Check sheet for the drawn part. Datum: minimum x, y, z corner. Units: mm. Give positions to 0.01 mm unless a question says otherwise; leave off trailing zeros. Write each loop counter-clockwise with the first axis right and the second up, starting at its lowest first coordinate (ties: lowest second). Pieces come first, ordered by that corner, then holes.
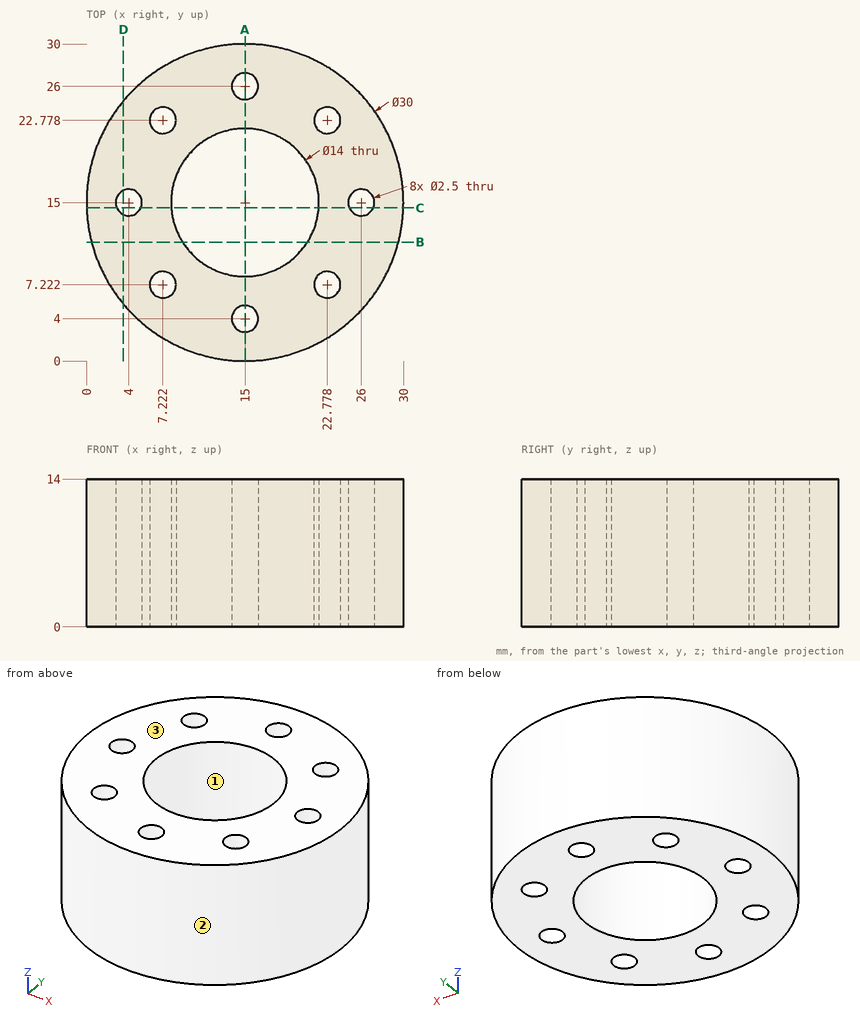
1) Sectioned sample at D-D on x = 3.5. Record the boundary of the cut face in (y, z).
2) Sectioned sample at C-C on y = 14.5. Record the boundary of the cut face in (x, z).
3) Sectioned sample at A-A on x = 15. Record the boundary of the cut face in (y, z), then the cut area to 3 significant figures.
4) Gauge pin test, flat ends, axial feed: pin 1 (2 mm diameter, centred on x = 4, y = 15, fed in from -Z); pin 2 (3 mm diameter, centred on y = 9.5, z = 9, fed in from -X); pin 3 (6 mm diameter, centred on y = 5, z = 1.5, fed in from +X); pin 4 (8 mm diameter, centred on y = 27, z = 11, fed in from -X). Record the tip position at first contact, or that the pin passes through.
5) Sectioned sample at B-B on y = 11.25. Record the boundary of the cut face in (x, z), then the cut area to 3 significant figures.
6) Scan lines: L1, parallel to Y at x = 15, z = 5; L2, parallel to Y at x = 7.5, z = 5.5; L3, parallel to X at y = 23, z = 9.75. Record each from-to range of solid material in increasing order.
7) Draft check along X on the marked faces 1, 2 and 3. Enter one of: +X half, -X half, draft (parallel to the pull), parting line (faces both ways), or undercut.
Answers below:
1. outline: (5.37, 0) - (13.85, 0) - (13.85, 14) - (5.37, 14) - close; (16.15, 0) - (24.63, 0) - (24.63, 14) - (16.15, 14) - close
2. outline: (0.01, 0) - (2.85, 0) - (2.85, 14) - (0.01, 14) - close; (5.15, 0) - (8.02, 0) - (8.02, 14) - (5.15, 14) - close; (21.98, 0) - (24.85, 0) - (24.85, 14) - (21.98, 14) - close; (27.15, 0) - (29.99, 0) - (29.99, 14) - (27.15, 14) - close
3. outline: (0, 0) - (2.75, 0) - (2.75, 14) - (0, 14) - close; (5.25, 0) - (8, 0) - (8, 14) - (5.25, 14) - close; (22, 0) - (24.75, 0) - (24.75, 14) - (22, 14) - close; (27.25, 0) - (30, 0) - (30, 14) - (27.25, 14) - close
3. area: 154 mm2
4. pin 1: passes through
4. pin 2: stops at x = 0.54
4. pin 3: stops at x = 28.27
4. pin 4: stops at x = 2.31
5. outline: (0.48, 0) - (9.09, 0) - (9.09, 14) - (0.48, 14) - close; (20.91, 0) - (29.52, 0) - (29.52, 14) - (20.91, 14) - close
5. area: 241 mm2
6. L1: y = 0 to 2.75, 5.25 to 8, 22 to 24.75, 27.25 to 30
6. L2: y = 2.01 to 6, 8.44 to 21.56, 24 to 27.99
6. L3: x = 2.31 to 5.99, 8.45 to 21.55, 24.01 to 27.69
7. face 1: undercut
7. face 2: parting line
7. face 3: draft
